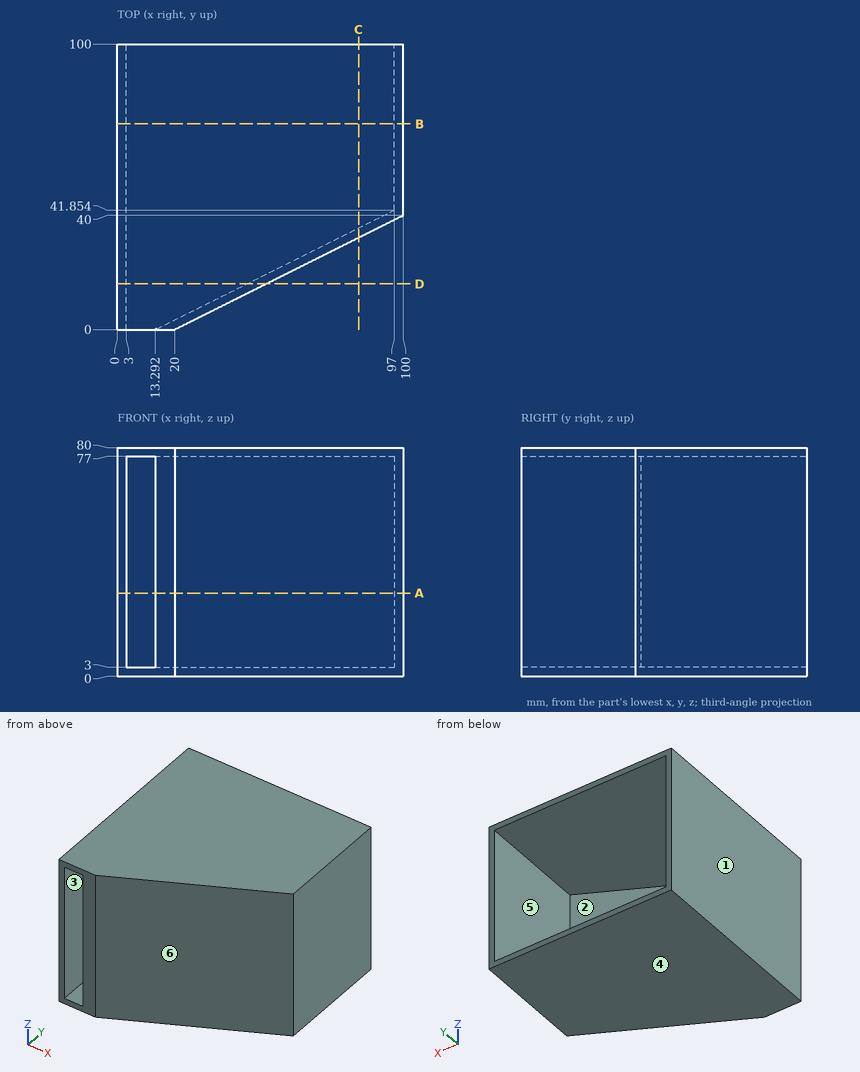
Study the drawing (mm; zero at the part's minimum x, y, z) and answer. A direction names the side the tool comes from. Round coordinates to 2 decimals unless told otherwise and drop trailing zeros. Loops run counter-clockwise (first coordinate to the right, second up) from the corner with the lowest first, then second, coordinate; pieces in that order, holes last.
Q1. Section A-A, the plane z = 29 is taken. Determine the outline of the cut face in (x, y), then the cut area to 3 significant figures.
Q2. Find the intervals of material crossed by line 1 (X direction, y = 80, z = 75.5); line 2 (Z direction, x = 38.5, y = 24); line 3 (X direction, y = 37, z = 62.5), in increasing order.
Q3. Which of the six approach directions +Z, -Z, +X, -X, +Y, -Y give full straight-line access (tool end or side, diameter ignored) to the marked faces 5 and 6?
Q4. Section B-B, the plane y = 72 is taken. Determine the outline of the cut face in (x, z), then the cut area to 3 significant figures.
Q5. Given pin 1 Ø2 at (x, z) = (22, 38) entering from -Y; pin 2 Ø4 at (x, z) = (76, 55.5) entering from +Y; pin 3 Ø4 at (y, z) = (30, 32) entering from +X, each flat-ended and moving along its own axis, determine where each tip first touches the part or whether it passes through.
Q6. For a pull along Z with two mould halves and no side action, classify the marked faces 1, 2, 3 and 4 as released by +Z, released by -Z, zero draft, split by the parting line, or undercut.
Q7. Section D-D, the plane y = 16 is taken. Determine the outline of the cut face in (x, z), then the cut area to 3 significant figures.
Q8. Section C-C, the plane x = 84.5 is taken. Determine the outline of the cut face in (y, z).
Completed:
1. outline: (0, 0) - (3, 0) - (3, 100) - (0, 100) - close; (13.29, 0) - (20, 0) - (100, 40) - (100, 100) - (97, 100) - (97, 41.85) - close
1. area: 752 mm2
2. line 1: x = 0 to 3, 97 to 100
2. line 2: z = 0 to 3, 77 to 80
2. line 3: x = 0 to 3, 87.29 to 94
3. face 5: +Y
3. face 6: +Z, -Z, +X, -Y
4. outline: (0, 0) - (100, 0) - (100, 80) - (0, 80) - close; hole (3, 3) - (97, 3) - (97, 77) - (3, 77) - close
4. area: 1,040 mm2
5. pin 1: stops at y = 0.5
5. pin 2: stops at y = 32.35
5. pin 3: stops at x = 84
6. face 1: zero draft
6. face 2: undercut
6. face 3: undercut
6. face 4: released by -Z
7. outline: (0, 0) - (52, 0) - (52, 80) - (0, 80) - close; hole (3, 3) - (45.29, 3) - (45.29, 77) - (3, 77) - close
7. area: 1,030 mm2
8. outline: (32.25, 0) - (100, 0) - (100, 3) - (35.6, 3) - (35.6, 77) - (100, 77) - (100, 80) - (32.25, 80) - close
